For this review, take the finished solid that the model builds, in its own axes (mm). A direction names the side the tool comes from. Give positions to 0.01 mm unless a question says otherwise; leave off trailing zeros. Order: outer loops, then holes, each group sorted by start corner. A loop starts at its lowest first (then second) coordinate and runs counter-clockwise, first axis right, second up.
from build123d import *

# Parameters (mm, degrees)
PAD002_DEPTH    = 1
POCKET002_DEPTH = 0.5
POCKET003_DEPTH = 0.25
POCKET004_DEPTH = 0.25
SKETCH009_W     = 8.5
SKETCH009_H     = 5
SKETCH009_W_2   = 11
PAD003_DEPTH    = 30
SKETCH010_R     = 4.05
SKETCH010_R_2   = 2.75
POCKET005_DEPTH = 54.281375499
SKETCH011_W     = 8
SKETCH011_H     = 3
SKETCH011_W_2   = 3
SKETCH011_H_2   = 8
PAD004_DEPTH    = 0.5
CHAMFER001_SIZE = 0.25
CHAMFER002_SIZE = 1


with BuildPart() as part:
    # Sketch005 (on Face1 of Binder) → Pad002 (new body)
    with BuildSketch(Plane(origin=(0, 0, -13), x_dir=(1, 0, 0), z_dir=(0, 0, -1))):
        Polygon((52, -58.333333), (40.686291501, -47.019624501), (-13.313708499, -47.019624501), (-13.313708499, -80.0117772123), (4, -110), (55, -110), (20.3427218622, -89.9906111378), align=None)
    extrude(amount=-PAD002_DEPTH)

    # Sketch006 (on Face8 of Pad002) → Pocket002 (cut)
    with BuildSketch(Plane(origin=(0, 0, -13), x_dir=(1, 0, 0), z_dir=(0, 0, -1))):
        Polygon((47.0856078708, -63.2477251292), (44.9289321881, -61.0910494466), (39.2013672605, -66.8186143742), (41.3580429431, -68.9752900569), align=None)
        Polygon((30.9846789191, -79.3486540809), (28.8280032365, -77.1919783983), (23.1004383089, -82.9195433259), (25.2571139915, -85.0762190085), align=None)
        Polygon((26.3615984185, -93.4656111378), (24.8365984185, -96.1069886193), (31.8514041892, -100.1569886193), (33.3764041892, -97.5156111378), align=None)
        Polygon((48.9811234437, -106.525), (41.966317673, -102.475), (40.441317673, -105.1163774815), (47.4561234437, -109.1663774815), align=None)
    extrude(amount=-POCKET002_DEPTH, mode=Mode.SUBTRACT)

    # Sketch007 (on Face5 of Pocket002) → Pocket003 (cut)
    with BuildSketch(Plane.XY.offset(-12)):
        Polygon((52, 58.333333), (40.686291501, 47.019624501), (-13.313708499, 47.019624501), (-13.313708499, 80.0117772123), (4, 110), (4.5773502692, 110), (-12.813708499, 79.8778026161), (-12.813708499, 47.519624501), (40.4791847198, 47.519624501), (51.6464466094, 58.6868863906), align=None)
    extrude(amount=-POCKET003_DEPTH, mode=Mode.SUBTRACT)

    # Sketch008 (on Face28 of Pocket003) → Pocket004 (cut)
    with BuildSketch(Plane.XY.offset(-12)):
        Polygon((20.3427218622, 89.9906111378), (2.8268236955, 79.8778026161), (-12.813708499, 79.8778026161), (-12.813708499, 79.3778026161), (2.9607982917, 79.3778026161), (20.708747266, 89.624585734), align=None)
    extrude(amount=-POCKET004_DEPTH, mode=Mode.SUBTRACT)

    # Sketch009 (on Face27 of Pocket004) → Pad003 (join)
    with BuildSketch(Plane.XY.offset(-12)):
        with Locations((19.106291501, 58.219624501)):
            Rectangle(SKETCH009_W, SKETCH009_H)
        with Locations((-4.803708499, 58.219624501)):
            Rectangle(SKETCH009_W_2, SKETCH009_H)
    extrude(amount=PAD003_DEPTH)

    # Sketch010 (on Face11 of Pad003) → Pocket005 (cut, through all)
    with BuildSketch(Plane.XZ.offset(-55.719624501)):
        with Locations((-4.803708499, 6.8)):
            Circle(SKETCH010_R)
        with Locations((19.106291501, 13.25)):
            Circle(SKETCH010_R_2)
    extrude(amount=-POCKET005_DEPTH, mode=Mode.SUBTRACT)

    # Sketch011 (on Face25 of Pocket005) → Pad004 (join)
    with BuildSketch(Plane(origin=(0, 0, -13), x_dir=(1, 0, 0), z_dir=(0, 0, -1))):
        with Locations((-5.313708499, -45.519624501)):
            Rectangle(SKETCH011_W, SKETCH011_H)
        with Locations((13.686291501, -45.519624501)):
            Rectangle(SKETCH011_W, SKETCH011_H)
        with Locations((32.686291501, -45.519624501)):
            Rectangle(SKETCH011_W, SKETCH011_H)
        with Locations((-14.813708499, -55.019624501)):
            Rectangle(SKETCH011_W_2, SKETCH011_H_2)
        with Locations((-14.813708499, -72.0117772123)):
            Rectangle(SKETCH011_W_2, SKETCH011_H_2)
        Polygon((-10.813708499, -84.3419042312), (-6.813708499, -91.2701074615), (-9.4117847103, -92.7701074615), (-13.4117847103, -85.8419042312), align=None)
        Polygon((-2.5, -98.7416697508), (-5.0980762114, -100.2416697508), (-1.0980762114, -107.1698729811), (1.5, -105.6698729811), align=None)
        Polygon((49.1715728753, -55.5049058753), (43.5147186258, -49.8480516258), (45.6360389693, -47.7267312822), (51.2928932188, -53.3835855317), align=None)
    extrude(amount=-PAD004_DEPTH)

    # Chamfer001
    chamfer001_edges = [part.edges().sort_by_distance(p)[0] for p in [
        (29.788675, 110, -12),
    ]]
    chamfer(chamfer001_edges, length=CHAMFER001_SIZE)

    # Chamfer002
    chamfer002_edges = [part.edges().sort_by_distance(p)[0] for p in [
        (-10.303708, 60.719625, 3),
        (-4.803708, 60.719625, 18),
        (0.696292, 60.719625, 3),
        (0.696292, 58.219625, 18),
        (-4.803708, 55.719625, 18),
        (-10.303708, 58.219625, 18),
        (14.856292, 60.719625, 3),
        (23.356292, 60.719625, 3),
        (19.106292, 60.719625, 18),
        (23.356292, 58.219625, 18),
        (19.106292, 55.719625, 18),
        (14.856292, 58.219625, 18),
        (-10.303708, 55.719625, 3),
        (0.696292, 55.719625, 3),
        (14.856292, 55.719625, 3),
        (23.356292, 55.719625, 3),
    ]]
    chamfer(chamfer002_edges, length=CHAMFER002_SIZE)


solid = part.part
1) We need section C-C on y = 104. Give the boundary of the cut face in (x, z), then the cut area to 3 significant figures.
Answer sheet:
outline: (-2.93, -13) - (41.09, -13) - (41.09, -12.5) - (44.61, -12.5) - (44.61, -12) - (1.11, -12) - (1.11, -12.25) - (0.54, -12.25) - (0.54, -12.5) - (-2.93, -12.5) - close
area: 43.9 mm2
2) Tool access review of faces 1 (the face through (-5, 45, -12.5)), 2 (the face through (-10, 88, -12.5)), 3 (the face through (47, 52, -12.5)): name each direction out of +Z, -Z, +X, -X, +Y, -Y from which nothing blocks a thin tool from reaching the whole face with its end or side.
Answer sheet:
face 1: +Z, +X, -X, -Y
face 2: +Z, -X, +Y
face 3: +Z, +X, -Y
3) Draft analysis for pull direction Y (two halves, no side actions). For faces 4 (the face through (-10.304, 58, 2)), 5 (the face through (42.11, 63.91, -12.75)), 6 (the face through (-5, 60.72, 2)), 7 (the face through (45, 106, -12.5)), state which applies: +Y half, -Y half, draft (parallel to the pull), parting line (faces both ways), or undercut.
Answer sheet:
face 4: draft
face 5: undercut
face 6: +Y half
face 7: undercut
4) Clearance check with flat-ended pins moving along their axes: pin 1 (0.9 mm diameter, centred on x = -15, y = 70.5, fed in from +Z); pin 2 (15 mm diameter, centred on x = 32.5, y = 89, fed in from +Z); pin 3 (0.6 mm diameter, centred on y = 46, z = -13, fed in from -X); pin 4 (4.5 mm diameter, centred on x = -4.5, z = 7.5, fed in from +Y). State where each tip first meets the part, or that it passes through.
Answer sheet:
pin 1: stops at z = -12.5
pin 2: stops at z = -12
pin 3: stops at x = -9.31
pin 4: passes through
5) We need section D-D on z = 13.25. Give the boundary of the cut face in (x, y).
Answer sheet:
outline: (-10.3, 56.72) - (-9.3, 55.72) - (-0.3, 55.72) - (0.7, 56.72) - (0.7, 59.72) - (-0.3, 60.72) - (-9.3, 60.72) - (-10.3, 59.72) - close; (14.86, 56.72) - (15.86, 55.72) - (16.36, 55.72) - (16.36, 60.72) - (15.86, 60.72) - (14.86, 59.72) - close; (21.86, 55.72) - (22.36, 55.72) - (23.36, 56.72) - (23.36, 59.72) - (22.36, 60.72) - (21.86, 60.72) - close
6) To check wall thickness, follow line 1 (X direction, y = 59, z = 2); line 2 (X direction, y = 57, z = 6); line 3 (Z direction, x = -12, y = 69.5). State the ranges of each line that lie inside material, in increasing order.
Answer sheet:
line 1: x = -10.3 to 0.7, 14.86 to 23.36
line 2: x = -10.3 to -8.77, -0.83 to 0.7, 14.86 to 23.36
line 3: z = -13 to -12
7) We need section B-B on x = 11. Give the boundary of the cut face in (y, z), then the cut area to 3 significant figures.
Answer sheet:
outline: (44.02, -13) - (110, -13) - (110, -12.25) - (109.75, -12) - (84.6, -12) - (84.6, -12.25) - (84.02, -12.25) - (84.02, -12) - (47.52, -12) - (47.52, -12.25) - (47.02, -12.25) - (47.02, -12.5) - (44.02, -12.5) - close
area: 64.2 mm2
8) We need section A-A on z = 6.8. Give the boundary of the cut face in (x, y).
Answer sheet:
outline: (-10.3, 56.72) - (-9.3, 55.72) - (-8.85, 55.72) - (-8.85, 60.72) - (-9.3, 60.72) - (-10.3, 59.72) - close; (-0.75, 55.72) - (-0.3, 55.72) - (0.7, 56.72) - (0.7, 59.72) - (-0.3, 60.72) - (-0.75, 60.72) - close; (14.86, 56.72) - (15.86, 55.72) - (22.36, 55.72) - (23.36, 56.72) - (23.36, 59.72) - (22.36, 60.72) - (15.86, 60.72) - (14.86, 59.72) - close
